from build123d import *

# Parameters (mm, degrees)
F0_R     = 37.5
F1_DEPTH = 10


with BuildPart() as f1:
    # F0 (on Top) → F1 (new body)
    with BuildSketch(Plane.XY):
        Circle(F0_R)
        with BuildLine():
            ThreePointArc((32.403703, 2.5), (32.475917, 1.250927), (32.5, 0))
            ThreePointArc((32.5, 0), (32.475917, -1.250927), (32.403703, -2.5))
            ThreePointArc((32.403703, -2.5), (22.98097, -22.98097), (2.5, -32.403703))
            ThreePointArc((2.5, -32.403703), (0, -32.5), (-2.5, -32.403703))
            ThreePointArc((-2.5, -32.403703), (-22.98097, -22.98097), (-32.403703, -2.5))
            ThreePointArc((-32.403703, -2.5), (-32.5, 0), (-32.403703, 2.5))
            ThreePointArc((-32.403703, 2.5), (-22.98097, 22.98097), (-2.5, 32.403703))
            ThreePointArc((-2.5, 32.403703), (0, 32.5), (2.5, 32.403703))
            ThreePointArc((2.5, 32.403703), (22.98097, 22.98097), (32.403703, 2.5))
        make_face(mode=Mode.SUBTRACT)
        with BuildLine():
            Line((2.5, 28.89204), (2.5, 32.403703))
            ThreePointArc((2.5, 32.403703), (0, 32.5), (-2.5, 32.403703))
            Line((-2.5, 32.403703), (-2.5, 28.89204))
            ThreePointArc((-2.5, 28.89204), (0, 29), (2.5, 28.89204))
        make_face()
        with BuildLine():
            ThreePointArc((32.403703, -2.5), (32.475917, -1.250927), (32.5, 0))
            ThreePointArc((32.5, 0), (32.475917, 1.250927), (32.403703, 2.5))
            Line((32.403703, 2.5), (28.89204, 2.5))
            ThreePointArc((28.89204, 2.5), (29, 0), (28.89204, -2.5))
            Line((28.89204, -2.5), (32.403703, -2.5))
        make_face()
        with BuildLine():
            ThreePointArc((-2.5, -32.403703), (0, -32.5), (2.5, -32.403703))
            Line((2.5, -32.403703), (2.5, -28.89204))
            ThreePointArc((2.5, -28.89204), (0, -29), (-2.5, -28.89204))
            Line((-2.5, -28.89204), (-2.5, -32.403703))
        make_face()
        with BuildLine():
            Line((-28.89204, 2.5), (-32.403703, 2.5))
            ThreePointArc((-32.403703, 2.5), (-32.5, 0), (-32.403703, -2.5))
            Line((-32.403703, -2.5), (-28.89204, -2.5))
            ThreePointArc((-28.89204, -2.5), (-29, 0), (-28.89204, 2.5))
        make_face()
    extrude(amount=-F1_DEPTH)


solid = f1.part
Source: CAD feature listing. Evaluate the final solid. Frame: model axes, mm. A direction names the side the tool comes from. Coordinates: 2 decimals unless noted, no trailing zeros. Loops run counter-clockwise (first coordinate to the right, second up) from the corner with the lowest first, then second, coordinate; pieces in that order, holes last. Notation, with made-up numbers: M 78.25,46 L 103.25,46 A17 ccw 103.25,57 Z; hole C -33,26.5 d3. An arc over 180 degrees is marked long. Answer in a Markdown table with one row per item.
Q1. Ray query, probe 1 along Y at (x, z) = (30, -2); probe 2 along Y at (x, z) = (13.5, -7); probe 3 along Y at (x, z) = (-11, -8.5). Return the intervals inside material, ascending. Write a range as from..to.
Answers below:
| item | result |
|---|---|
| probe 1 | y = -22.5..-12.5, -2.5..2.5, 12.5..22.5 |
| probe 2 | y = -34.99..-29.56, 29.56..34.99 |
| probe 3 | y = -35.85..-30.58, 30.58..35.85 |
Q2. Draft query along Y for faces 3 (the flat face through (0, 31, -10)), 4 (the cylindrical face through (-23.21, 22.75, -4.93)), 5 (the cylindrical face through (-4.88, 37.18, -4.93)). Return one class per face: pulls with the +Y half, pulls with the -Y half, needs draft (parallel to the pull), parting line crosses it, or undercut.
Answers below:
| item | result |
|---|---|
| face 3 | needs draft |
| face 4 | undercut |
| face 5 | parting line crosses it |
Q3. Set-up query: faces 1 (the cylindrical face through (23.21, -22.75, -4.93)), 2 (the flat face through (0, 31, 0)). Return all of +Z, -Z, +X, -X, +Y, -Y with unobstructed straight access to the full face (end or side cutting, diameter ignored); none if empty.
Answers below:
| item | result |
|---|---|
| face 1 | +Z, -Z |
| face 2 | +Z, +X, -X, +Y, -Y |
Q4. First-contact query: pin 1 (1 mm diameter, centred on x = 28.5, z = -1.5, fed in from +Y); pin 2 (1.1 mm diameter, centred on y = -31, z = -6, fed in from -X); pin 3 (2 mm diameter, centred on y = -15, z = -4.5, fed in from +X); pin 4 (1.5 mm diameter, centred on x = -29, y = -16, fed in from +Z). Flat tips, straight axial feed; report the tip coordinate or a pass-through.
Answers below:
| item | result |
|---|---|
| pin 1 | stops at y = 24.94 |
| pin 2 | stops at x = -21.89 |
| pin 3 | stops at x = 34.79 |
| pin 4 | stops at z = 0 |
Q5. Section C-C on x = -30. Return the cut outline in (y, z), plus the area to 3 significant figures.
Answers below:
| item | result |
|---|---|
| outline | M -22.5,-10 L -12.5,-10 L -12.5,0 L -22.5,0 Z; M -2.5,-10 L 2.5,-10 L 2.5,0 L -2.5,0 Z; M 12.5,-10 L 22.5,-10 L 22.5,0 L 12.5,0 Z |
| area | 250 mm^2 |
Q6. Section D-D on z = -2.25. Return the cut outline in (x, y).
Answers below:
| item | result |
|---|---|
| outline | C 0,0 d75; hole M -32.4,-2.5 A32.5 ccw -2.5,-32.4 L -2.5,-28.89 A29 ccw 2.5,-28.89 L 2.5,-32.4 A32.5 ccw 32.4,-2.5 L 28.89,-2.5 A29 ccw 28.89,2.5 L 32.4,2.5 A32.5 ccw 2.5,32.4 L 2.5,28.89 A29 ccw -2.5,28.89 L -2.5,32.4 A32.5 ccw -32.4,2.5 L -28.89,2.5 A29 ccw -28.89,-2.5 Z |
Q7. Section A-A on x = 0. Return the cut outline in (y, z).
Answers below:
| item | result |
|---|---|
| outline | M -37.5,-10 L -29,-10 L -29,0 L -37.5,0 Z; M 29,-10 L 37.5,-10 L 37.5,0 L 29,0 Z |
